Here's how the part is built. I have some questions about the finished solid (model axes, mm). Face numbers are marked on the shaded views. A direction names the side the tool comes from. Give positions to 0.01 mm unless a question says otherwise; leave off trailing zeros. Write each loop counter-clockwise with the first axis right and the second up, starting at its lowest first coordinate (ties: lowest second). Pieces come first, ordered by that corner, then holes. Notation, with made-up numbers: (76.25, -7) -> (86.25, -7) arc R15 cw to (86.25, 16) -> close; hole circle Ø3 at (47, 39). An arc over 180 degrees is marked (long way). Return JSON: item names as keys, results as strings.
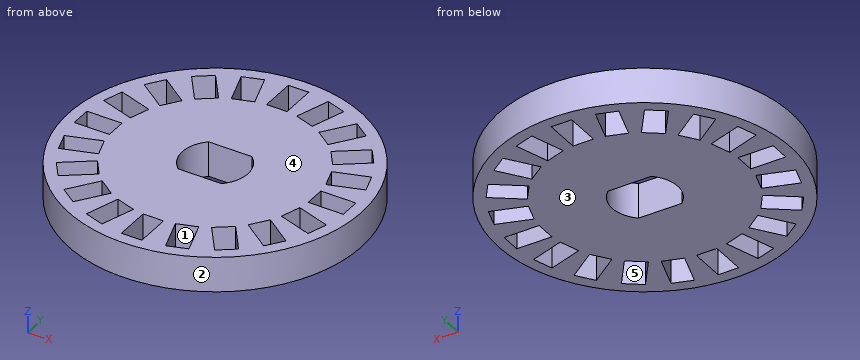
Autodesk Inventor part; units mm, degrees
ref_plane "YZ Plane" through (0, 0, 0) normal (1, 0, 0) x (0, 1, 0)
ref_plane "XZ Plane" through (0, 0, 0) normal (0, 1, 0) x (-1, 0, 0)
ref_plane "XY Plane" through (0, 0, 0) normal (0, 0, 1) x (1, 0, 0)
sketch "Boceto1" plane through (0, 0, 0) normal (0, 0, 1) x (1, 0, 0)
  circle A0 centre (0, 0) radius 12.5
  circle A1 centre (0, 0) radius 2.8
  line L0 (-1.852, 2.1) -> (1.852, 2.1)
  line L1 (-1.852, -2.1) -> (1.852, -2.1)
  dimension "d0" = 25
  dimension "d1" = 5.6
  dimension "d2" = 2.1
  dimension "d3" = 2.1
extrude "Extrusión1" add sketch "Boceto1" along normal blind 3 contours A0 | L0 A1 | A1 L1
sketch "Boceto2" plane through (0, 0, 3) normal (0, 0, 1) x (1, 0, 0)
  line L0 (-0.875, 11.5) -> (0.875, 11.5)
  line L1 (0.875, 11.5) -> (0.875, 8.5)
  line L2 (0.875, 8.5) -> (-0.875, 8.5)
  line L3 (-0.875, 8.5) -> (-0.875, 11.5)
  point P0 (0, 0)
  point P1 (0, 11.5)
  dimension "d6" = 3
  dimension "d7" = 1.75
  dimension "d8" = 8.5
extrude "Extrusión2" cut sketch "Boceto2" against normal through all
pattern_circular "Patrón circular1" count 20 over 360 about axis through (0, 0, -10) along (0, 0, 1) of "Extrusión2"
properties part number "Disco_encoder"
1. Suppose I cut it at C-C, the plane y = 7. List the corners of the cut face in (x, z) for me, and give its area (3 significant figures).
Taken from the geometry:
{"outline": "(-10.36, 0) -> (-9.13, 0) -> (-9.13, 3) -> (-10.36, 3) -> close; (-8.15, 0) -> (-6.17, 0) -> (-6.17, 3) -> (-8.15, 3) -> close; (-4.83, 0) -> (4.83, 0) -> (4.83, 3) -> (-4.83, 3) -> close; (6.17, 0) -> (8.15, 0) -> (8.15, 3) -> (6.17, 3) -> close; (9.13, 0) -> (10.36, 0) -> (10.36, 3) -> (9.13, 3) -> close", "area": "48.2 mm²"}
2. Suppose I cut it at B-B, the plane x = 0. List the corners of the cut face in (y, z) for me, and give its area (3 significant figures).
Taken from the geometry:
{"outline": "(-12.5, 0) -> (-11.5, 0) -> (-11.5, 3) -> (-12.5, 3) -> close; (-8.5, 0) -> (-2.1, 0) -> (-2.1, 3) -> (-8.5, 3) -> close; (2.1, 0) -> (8.5, 0) -> (8.5, 3) -> (2.1, 3) -> close; (11.5, 0) -> (12.5, 0) -> (12.5, 3) -> (11.5, 3) -> close", "area": "44.4 mm²"}
3. If I drill on line 1 (Y direction, x = -5.25, z = 1.65); line 2 (X direction, y = 10, z = 2.05) (3 decimals); line 3 (Y direction, x = 4.5, z = 2.35), over which ranges is the centre line in solid material (lowest first)? Write a range as [from, to].
Taken from the geometry:
{"line 1": "y = [-11.34, -8.71], [-6.69, 6.69], [8.71, 11.34]", "line 2": "x = [-7.5, -4.169], [-2.329, -0.875], [0.875, 2.329], [4.169, 7.5]", "line 3": "y = [-11.66, -7.68], [-7.24, 7.24], [7.68, 11.66]"}
4. Suppose I cut it at A-A, the plane y = 0. List the corners of the cut face in (x, z) for me, and give its area (3 significant figures).
Taken from the geometry:
{"outline": "(-12.5, 0) -> (-11.5, 0) -> (-11.5, 3) -> (-12.5, 3) -> close; (-8.5, 0) -> (-2.8, 0) -> (-2.8, 3) -> (-8.5, 3) -> close; (2.8, 0) -> (8.5, 0) -> (8.5, 3) -> (2.8, 3) -> close; (11.5, 0) -> (12.5, 0) -> (12.5, 3) -> (11.5, 3) -> close", "area": "40.2 mm²"}
5. If we mould it in two halves opening along X, with no side actions, what happens to the marked faces 1, 2 and 3? For each: released by +X, released by -X, zero draft, split by the parting line, or undercut.
Taken from the geometry:
{"face 1": "undercut", "face 2": "split by the parting line", "face 3": "zero draft"}
6. Which directions (+Z, -Z, +X, -X, +Y, -Y) give clear straight access to the entire face, cutting with the end or side of a thin tool? Please do the marked faces 4 and 5.
Taken from the geometry:
{"face 4": "+Z, +X, -X, +Y, -Y", "face 5": "+Z, -Z"}
7. For pin 1 Ø1.5 at (x, z) = (10, 1) entering from +Y; pin 2 Ø1 at (y, z) = (-4, 2.5) entering from -X; pin 3 Ø1.5 at (y, z) = (9.5, 1) entering from +X; pin 4 Ø0.9 at (x, z) = (0.5, 1) entering from +Y, each with a flat end and sliding along its axis, tell me the tip position at first contact or that it passes through.
Taken from the geometry:
{"pin 1": "stops at y = 8.41", "pin 2": "stops at x = -12", "pin 3": "stops at x = 8.93", "pin 4": "stops at y = 12.5"}
8. Suppose I cut it at D-D, the plane z = 0.5. Count the separate pieces of the cut face and the enclosed holes in it, and give its area (3 significant figures).
Taken from the geometry:
{"separate pieces": "1", "enclosed holes": "21", "area": "365 mm²"}
